```python
from build123d import *

# Parameters (mm, degrees)
F0_R     = 2.5
F1_DEPTH = 2


with BuildPart() as f1:
    # F0 (on Front) → F1 (new body)
    with BuildSketch(Plane.XZ):
        with BuildLine():
            add(Edge.make_bspline(
                [(5, 0), (4.926064, -0.492134), (4.853598, -0.978139), (4.782619, -1.458273)],
                knots=[0, 0, 0, 0, 1.163643, 1.163643, 1.163643, 1.163643], degree=3))
            ThreePointArc((5, 0), (0, 5), (-5, 0))
            add(Edge.make_bspline(
                [(-5, 0), (-4.926064, -0.492134), (-4.853598, -0.978139), (-4.782619, -1.458273)],
                knots=[0, 0, 0, 0, 1.163643, 1.163643, 1.163643, 1.163643], degree=3))
            ThreePointArc((-4.782619, -1.458273), (0, -5), (4.782619, -1.458273))
        make_face()
        Circle(F0_R, mode=Mode.SUBTRACT)
        with BuildLine():
            ThreePointArc((4.782619, -1.458273), (4.945356, -0.737193), (5, 0))
            add(Edge.make_bspline(
                [(5, 0), (4.926064, -0.492134), (4.853598, -0.978139), (4.782619, -1.458273)],
                knots=[0, 0, 0, 0, 1.163643, 1.163643, 1.163643, 1.163643], degree=3))
        make_face()
        with BuildLine():
            add(Edge.make_bspline(
                [(-5, 0), (-4.926064, -0.492134), (-4.853598, -0.978139), (-4.782619, -1.458273)],
                knots=[0, 0, 0, 0, 1.163643, 1.163643, 1.163643, 1.163643], degree=3))
            ThreePointArc((-5, 0), (-4.945356, -0.737193), (-4.782619, -1.458273))
        make_face()
        with BuildLine():
            add(Edge.make_bspline(
                [(4.782619, -1.458273), (1.891675, -21.013817), (1.467811, -30.83033), (4.740109, -48.408974)],
                knots=[1.163643, 1.163643, 1.163643, 1.163643, 48.558084, 48.558084, 48.558084, 48.558084], degree=3))
            ThreePointArc((4.782619, -1.458273), (0, -5), (-4.782619, -1.458273))
            add(Edge.make_bspline(
                [(-4.782619, -1.458273), (-1.891675, -21.013817), (-1.467811, -30.83033), (-4.740109, -48.408974)],
                knots=[1.163643, 1.163643, 1.163643, 1.163643, 48.558084, 48.558084, 48.558084, 48.558084], degree=3))
            ThreePointArc((-4.740109, -48.408974), (0, -45), (4.740109, -48.408974))
        make_face()
        with BuildLine():
            add(Edge.make_bspline(
                [(4.740109, -48.408974), (4.82229, -48.850442), (4.906801, -49.296806), (4.993663, -49.748342)],
                knots=[48.558084, 48.558084, 48.558084, 48.558084, 49.748343, 49.748343, 49.748343, 49.748343], degree=3))
            ThreePointArc((4.740109, -48.408974), (0, -45), (-4.740109, -48.408974))
            add(Edge.make_bspline(
                [(-4.740109, -48.408974), (-4.82229, -48.850442), (-4.906801, -49.296806), (-4.993663, -49.748342)],
                knots=[48.558084, 48.558084, 48.558084, 48.558084, 49.748343, 49.748343, 49.748343, 49.748343], degree=3))
            ThreePointArc((-4.993663, -49.748342), (-0.125869, -54.998415), (5, -50))
            ThreePointArc((5, -50), (4.998415, -49.874131), (4.993663, -49.748342))
        make_face()
        with Locations((0, -50)):
            Circle(F0_R, mode=Mode.SUBTRACT)
        with BuildLine():
            ThreePointArc((4.993663, -49.748342), (4.912744, -49.069977), (4.740109, -48.408974))
            add(Edge.make_bspline(
                [(4.740109, -48.408974), (4.82229, -48.850442), (4.906801, -49.296806), (4.993663, -49.748342)],
                knots=[48.558084, 48.558084, 48.558084, 48.558084, 49.748343, 49.748343, 49.748343, 49.748343], degree=3))
        make_face()
        with BuildLine():
            add(Edge.make_bspline(
                [(-4.740109, -48.408974), (-4.82229, -48.850442), (-4.906801, -49.296806), (-4.993663, -49.748342)],
                knots=[48.558084, 48.558084, 48.558084, 48.558084, 49.748343, 49.748343, 49.748343, 49.748343], degree=3))
            ThreePointArc((-4.740109, -48.408974), (-4.912744, -49.069977), (-4.993663, -49.748342))
        make_face()
    extrude(amount=F1_DEPTH)


solid = f1.part
```
Could you check a few things on this model? Use its own coordinates, in mm. A direction names the side the tool comes from. Round coordinates to 2 decimals unless told otherwise and drop trailing zeros. Loops run counter-clockwise (first coordinate to the right, second up) from the corner with the lowest first, then second, coordinate; pieces in that order, holes last. Notation, with made-up numbers: M 16,76 L 55,76 A27 ccw 55,106 Z; hole C 76,-15.5 d4. An arc over 180 degrees is marked long. Put each result on its own line as item: value.
Q1. Imagine slicing it at A-A (x = 0). Write out the boundary of the cut face in (y, z).
Check result:
outline: M -2,-55 L 0,-55 L 0,-52.5 L -2,-52.5 Z; M -2,-47.5 L 0,-47.5 L 0,-2.5 L -2,-2.5 Z; M -2,2.5 L 0,2.5 L 0,5 L -2,5 Z
Q2. On a 3-axis mill with a long thin cutter (end or side, diameter ignored), from which of +Z, -Z, +X, -X, +Y, -Y can I reach the whole of each face in a straight line? I mean faces 1 (the face through (-4.91, -0.99, -49.06)), 2 (the face through (4.944, -0.986, -0.747)), 3 (the face through (-0.54, -0.99, -52.44)). Say none if no direction works.
Check result:
face 1: -X, +Y, -Y
face 2: +X, +Y, -Y
face 3: +Y, -Y
Q3. For pin 1 (3 mm diameter, centred on x = -1, z = -28.5, fed in from +Y), with a flat end and sliding along its axis, tell me the tip position at first contact or that it passes through.
Check result:
pin 1: y = 0
Q4. I need wall thicknesses on probe 1 along Z at (x, y) = (0, -0.75); probe 2 along Z at (x, y) = (0.5, -1.05); probe 3 along X at (y, z) = (-1.8, -29.5). Which ranges of each line are inside material? Lowest first, please.
Check result:
probe 1: -55 to -52.5, -47.5 to -2.5, 2.5 to 5
probe 2: -54.97 to -52.45, -47.55 to -2.45, 2.45 to 4.97
probe 3: -2.49 to 2.49
Q5. Thinking about a two-plate mould opening in X: for faces 4 (the face through (0, -1, -55)), 5 (the face through (-0.54, -0.99, -2.44)), 6 (the face through (0, -2, -25)), 7 (the face through (4.915, -0.986, -49.079)), which applies, released by +X, released by -X, zero draft, split by the parting line, or undercut?
Check result:
face 4: split by the parting line
face 5: undercut
face 6: zero draft
face 7: released by +X
Q6. Imagine slicing it at B-B (y = -0.8). State how many separate pieces and enclosed holes the cut face has, then the cut area to 3 significant figures.
Check result:
separate pieces: 1
enclosed holes: 2
area: 377 mm2
